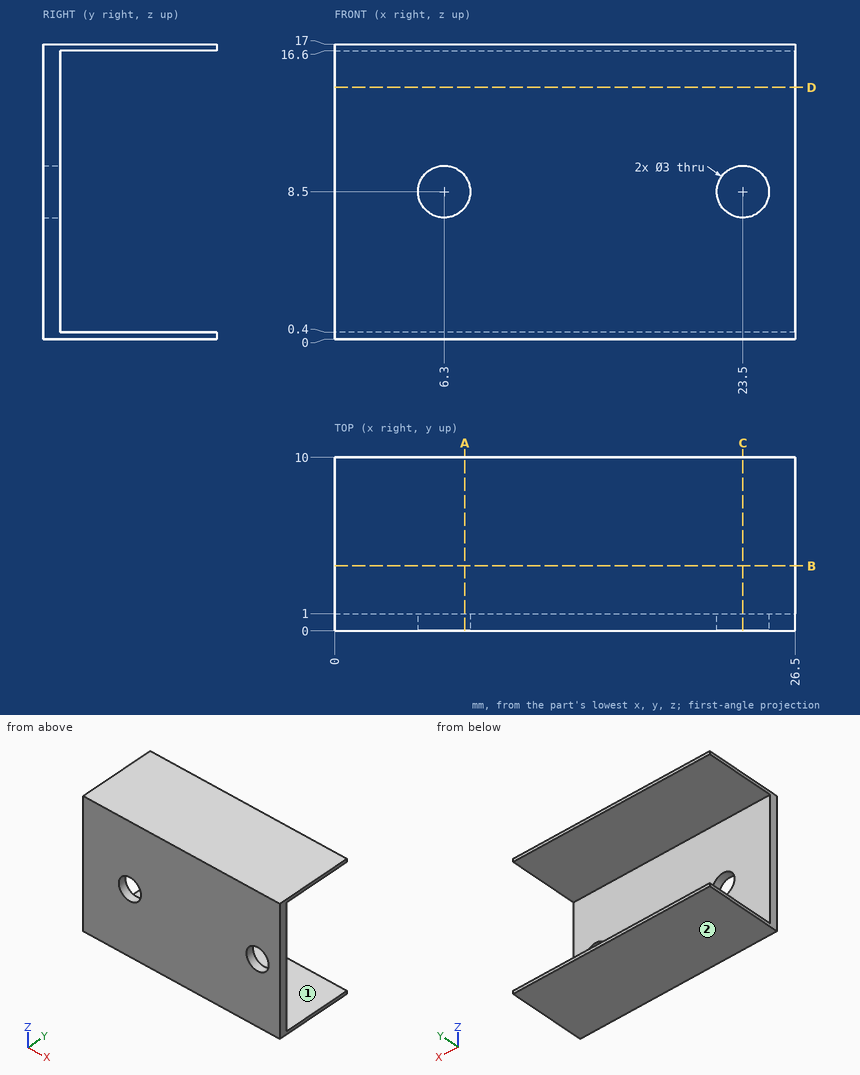
Job drawing, mm, ordinate dimensions from the low corner. One solid piece. A direction names the side the tool comes from. Give positions to 0.01 mm unless a question says otherwise; leave off trailing zeros. Order: outer loops, then holes, each group sorted by start corner. A loop starts at its lowest first (then second) coordinate and runs counter-clockwise, first axis right, second up. Notation, with made-up numbers: (63.25, 81.5) - (110.25, 81.5) arc R27 cw to (110.25, 101.5) - close; hole circle Ø2 at (0, 44). An arc over 180 degrees is marked (long way). One line per question, with ' | ' between items.
1. Which spindle directions (+Z, -Z, +X, -X, +Y, -Y) get a long thin tool onto all of the face, cutting with end or side? Do the marked faces 1 and 2. Say none if no direction does.
Filled in:
face 1: +X, -X, +Y | face 2: -Z, +X, -X, +Y, -Y
2. Band-saw the part on C-C on x = 23.5. List the corners of the cut face in (y, z).
Filled in:
outline: (0, 0) - (10, 0) - (10, 0.4) - (1, 0.4) - (1, 7) - (0, 7) - close; (0, 10) - (1, 10) - (1, 16.6) - (10, 16.6) - (10, 17) - (0, 17) - close
3. Band-saw the part on A-A on x = 7.5. List the corners of the cut face in (y, z), then the cut area to 3 significant figures.
Filled in:
outline: (0, 0) - (10, 0) - (10, 0.4) - (1, 0.4) - (1, 7.6) - (0, 7.6) - close; (0, 9.4) - (1, 9.4) - (1, 16.6) - (10, 16.6) - (10, 17) - (0, 17) - close | area: 22.4 mm²
4. Drop a flat-ended pin along its axis: P1, Ø2, axis at x = 10, z = 6.5, coming from the +Y side. Give the stop position or say it passes through.
Filled in:
P1: y = 1
5. Drill centre lines: probe 1 along X at (y, z) = (0.45, 8.5); probe 2 along Z at (x, y) = (6.75, 3.5); probe 3 along Z at (x, y) = (23.5, 0.75). Where is each one in solid material? Low to high.
Filled in:
probe 1: 0 to 4.8, 7.8 to 22, 25 to 26.5 | probe 2: 0 to 0.4, 16.6 to 17 | probe 3: 0 to 7, 10 to 17
6. Band-saw the part on D-D on z = 14.5. List the corners of the cut face in (x, y).
Filled in:
outline: (0, 0) - (26.5, 0) - (26.5, 1) - (0, 1) - close
7. Band-saw the part on B-B on y = 3.75. List the corners of the cut face in (x, z).
Filled in:
outline: (0, 0) - (26.5, 0) - (26.5, 0.4) - (0, 0.4) - close; (0, 16.6) - (26.5, 16.6) - (26.5, 17) - (0, 17) - close
